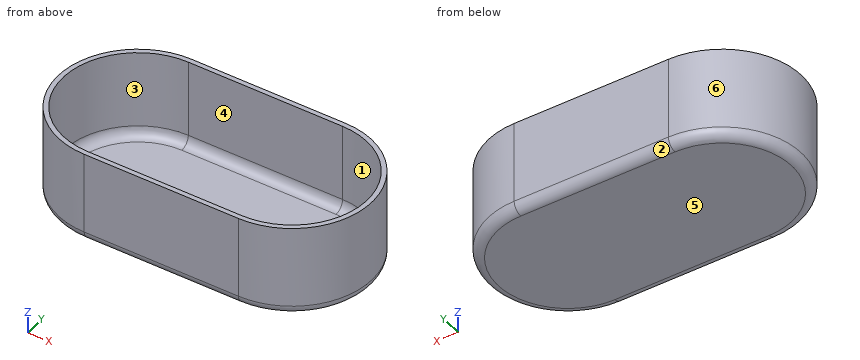
from build123d import *

# Parameters (mm, degrees)
PAD003_DEPTH   = 19
THICKNESS001_T = -1
FILLET004_R    = 2
FILLET005_R    = 2


with BuildPart() as part:
    # Sketch008 → Pad003 (new body)
    with BuildSketch(Plane.XY):
        with BuildLine():
            ThreePointArc((-83, 72.5), (-99.5, 56), (-83, 39.5))
            Line((-83, 39.5), (-50.5, 39.5))
            ThreePointArc((-50.5, 39.5), (-34, 56), (-50.5, 72.5))
            Line((-50.5, 72.5), (-83, 72.5))
        make_face()
    extrude(amount=PAD003_DEPTH)

    # Thickness001
    thickness001_openings = [part.faces().sort_by_distance(p)[0] for p in [
        (-66.75, 56, 19),
    ]]
    offset(amount=THICKNESS001_T, openings=thickness001_openings)

    # Fillet004
    fillet004_edges = [part.edges().sort_by_distance(p)[0] for p in [
        (-98.5, 56, 1),
        (-66.75, 40.5, 1),
        (-35, 56, 1),
        (-66.75, 71.5, 1),
    ]]
    fillet(fillet004_edges, radius=FILLET004_R)

    # Fillet005
    fillet005_edges = [part.edges().sort_by_distance(p)[0] for p in [
        (-99.5, 56, 0),
        (-66.75, 39.5, 0),
        (-34, 56, 0),
        (-66.75, 72.5, 0),
    ]]
    fillet(fillet005_edges, radius=FILLET005_R)


with BuildPart() as part_1:
    # Body003 placement: moved
    add(part.part.moved(Location((233, -61, 49))))


solid = part_1.part
Geometry check sheet. Reference: the model listing, model coordinates, mm. Face numbers are marked on the shaded views. A direction names the side the tool comes from. Give positions to 0.01 mm unless a question says otherwise; leave off trailing zeros. Write each loop counter-clockwise with the first axis right and the second up, starting at its lowest first coordinate (ties: lowest second). Pieces come first, ordered by that corner, then holes. Notation, with made-up numbers: M -38.75,16 L -30.75,16 A25 ccw -30.75,41 Z; hole C 57.25,31 d6. An arc over 180 degrees is marked long. One line per question, with ' | ' between items.
1. Scan lines: line 1 along Y through (x, z) = (182, 64); line 2 along Z through (x, y) = (163, -1.5); line 3 along X through (y, z) = (-5, 62.5). Record each from-to range of solid material in increasing order. Write a range as from..to.
Ans:
line 1: -21.5..-20.5, 10.5..11.5 | line 2: 49..50 | line 3: 133.5..134.5, 198..199
2. Gauge pin test, flat end, axial feed: pin 1 (10 mm diameter, centred on x = 185.5, y = -8.5, fed in from +Z). Record the tip position at first contact, or that the pin passes through.
Ans:
pin 1: z = 50
3. Set-up check for the marked faces 1 and 2: record each of +Z, -Z, +X, -X, +Y, -Y from which the full face is reachable in a straight line by a thin tool's end or side.
Ans:
face 1: +Z | face 2: -Z, +X, -X, +Y
4. Cross-section at C-C (y = -5). Enter the section's corners in (x, z).
Ans:
outline: M 133.5,51 A2 ccw 135.5,49 L 197,49 A2 ccw 199,51 L 199,68 L 198,68 L 198,52 A2 cw 196,50 L 136.5,50 A2 cw 134.5,52 L 134.5,68 L 133.5,68 Z
5. Cross-section at A-A (z = 66.75). Enter the section's corners in (x, y), plus the area to 3 significant figures.
Ans:
outline: M 150,-21.5 L 182.5,-21.5 A16.5 ccw 182.5,11.5 L 150,11.5 A16.5 ccw Z; hole M 150,-20.5 L 182.5,-20.5 A15.5 ccw 182.5,10.5 L 150,10.5 A15.5 ccw Z | area: 166 mm2
6. Cross-section at B-B (x = 179). Enter the section's corners in (y, z), plus the area to 3 significant figures.
Ans:
outline: M -21.5,51 A2 ccw -19.5,49 L 9.5,49 A2 ccw 11.5,51 L 11.5,68 L 10.5,68 L 10.5,52 A2 cw 8.5,50 L -18.5,50 A2 cw -20.5,52 L -20.5,68 L -21.5,68 Z | area: 69.0 mm2
7. Mould release check, pull along X, two halves, no side actions. Record for the marked faces 3, 4, 5 and 6: released by +X, released by -X, zero draft, split by the parting line, or undercut.
Ans:
face 3: undercut | face 4: undercut | face 5: zero draft | face 6: released by -X
